Geometry: final body of the model. Coordinates: model frame, mm. A direction names the side the tool comes from. Coordinates: 2 decimals unless noted, no trailing zeros. Order: outer loops, then holes, each group sorted by start corner. A loop starts at its lowest first (then second) coordinate and runs counter-clockwise, first axis right, second up. Notation, with made-up numbers: M 34,-4.75 L 66,-4.75 A20 ccw 66,5.25 Z; hole C 78,-26.5 d2. An arc over 180 degrees is marked long. Use CSV: the item, a comma, the result in double quotes. Start each with the question number.
Q1. Access query for faces 5 (the face through (19.72, 57.1, -140.08)), 6 (the face through (14.58, 202.24, -189)). Directions: +Z, -Z, +X, -X, +Y, -Y. A direction counts if a zero-diameter tool reaches every point of the face in a straight line with its end or side. Return the directions, or none.
Q2. Ray query, probe 1 along X at (y, z) = (4.5, -30); probe 2 along Y at (x, z) = (7.5, -17); probe 3 along Z at (x, y) = (38, 210.5). Return the intervals inside material, ascending.
Q3. First-contact query: P1, Ø7, axis at x = 30, y = 217, coming from the +Z side; P2, Ø10, axis at x = 35.5, y = 45, coming from the -Z side; P3, Ø4, axis at x = 26.5, y = 29.5, coming from the +Z side. Flat tips, straight axial feed; report the tip coordinate or a pass-through.
Q4. Mould query, pull axis Y, two halves, no side actions, for faces 1 (the face through (10.001, 202.684, -184.437)), 2 (the face through (32.027, 7.383, -31.859)), 3 (the face through (23.47, 171.38, -192.04)), 4 (the face through (20, 0, -20)). Classes: +Y half, -Y half, draft (parallel to the pull), parting line (faces both ways), or undercut.
Q5. Section query B-B, the plane y = 187. Output: boundary loops of the cut face in (x, z), and give its area (3 significant figures).
Q6. Section query D-D, the plane y = 39.5. Output: boundary loops of the cut face in (x, z), and give its area (3 significant figures).
Q7. Section query A-A, the plane x = 20. Output: boundary loops of the cut face in (y, z), and give its area (3 significant figures).
Q8. Section query C-C, the plane z = -37. Output: boundary loops of the cut face in (x, y).
from build123d import *

# Parameters (mm, degrees)
BOSS_EXTRUDE2_DEPTH            = 40
M5_CLEARANCE_HOLE2_D           = 5.5
M5_CLEARANCE_HOLE2_CSINK_D     = 5.55
M5_CLEARANCE_HOLE2_CSINK_ANGLE = 90
CUT_EXTRUDE1_REACH             = 303.917
SKETCH10_R                     = 16
SKETCH11_R                     = 18.6
CUT_EXTRUDE2_DEPTH             = 9
FILLET1_START                  = -1
FILLET1_DEPTH                  = 218.778561538
FILLET1_START_2                = -196
FILLET1_2_DEPTH                = 188.2945
M5_CLEARANCE_HOLE3_D           = 5.5
M5_CLEARANCE_HOLE3_CSINK_D     = 5.55
M5_CLEARANCE_HOLE3_CSINK_ANGLE = 90


with BuildPart() as part:
    # Sketch6 → Boss-Extrude2 (new body)
    with BuildSketch(Plane(origin=(0, 0, 0), x_dir=(0, 0, -1), z_dir=(1, 0, 0))):
        with BuildLine():
            Line((0, 0), (40, 0))
            ThreePointArc((40, 0), (149.601551084, 45.398448916), (195, 155))
            Line((195, 155), (195, 227))
            Line((195, 227), (180, 227))
            Line((180, 227), (180, 155))
            ThreePointArc((180, 155), (138.994949366, 56.005050634), (40, 15))
            Line((40, 15), (0, 15))
            Line((0, 15), (0, 0))
        make_face()
    extrude(amount=BOSS_EXTRUDE2_DEPTH)

    # M5 Clearance Hole2 (through all)
    with Locations(Plane(origin=(0, 15, 0), x_dir=(1, 0, 0), z_dir=(0, 1, 0))):
        with Locations((10, 30), (30, 30), (10, 10), (30, 10)):
            CounterSinkHole(M5_CLEARANCE_HOLE2_D / 2, M5_CLEARANCE_HOLE2_CSINK_D / 2, counter_sink_angle=M5_CLEARANCE_HOLE2_CSINK_ANGLE)

    # Sketch10 → Cut-Extrude1 (cut, up to next)
    with BuildSketch(Plane(origin=(0, 0, -195), x_dir=(-1, 0, 0), z_dir=(0, 0, -1)), mode=Mode.PRIVATE) as cut_extrude1_sk1:
        with Locations((-20, 187)):
            Circle(SKETCH10_R)
    cut_extrude1_tool1 = extrude(cut_extrude1_sk1.sketch, amount=-CUT_EXTRUDE1_REACH, mode=Mode.PRIVATE) & part.part
    add(cut_extrude1_tool1.solids().sort_by_distance((20, 187, -195))[0], mode=Mode.SUBTRACT)

    # Sketch11 → Cut-Extrude2 (cut)
    with BuildSketch(Plane(origin=(0, 0, -180), x_dir=(-1, 0, 0), z_dir=(0, 0, -1))):
        with Locations((-20, 187)):
            Circle(SKETCH11_R)
    extrude(amount=CUT_EXTRUDE2_DEPTH, mode=Mode.SUBTRACT)

    # Fillet1: read off the stored shape, not the designer's step
    # Fillet1 outline → Fillet1 (cut)
    with BuildSketch(Plane(origin=(0, 0, 0), x_dir=(1, 0, 0), z_dir=(0, 1, 0)).offset(FILLET1_START)):
        with BuildLine():
            Line((40, 0), (40, 10))
            add(Edge.make_bspline(
                [(40, 10), (40, 0), (30, 0)],
                knots=[0, 0, 0, 1, 1, 1], degree=2, weights=[1, 0.707106781, 1]))
            Line((30, 0), (40, 0))
        make_face()
        with BuildLine():
            Line((0, 0), (10, 0))
            add(Edge.make_bspline(
                [(10, 0), (0, 0), (0, 10)],
                knots=[0, 0, 0, 1, 1, 1], degree=2, weights=[1, 0.707106781, 1]))
            Line((0, 10), (0, 0))
        make_face()
    extrude(amount=FILLET1_DEPTH, mode=Mode.SUBTRACT)

    # Fillet1 2 outline → Fillet1 2 (cut)
    with BuildSketch(Plane.XY.offset(FILLET1_START_2)):
        with BuildLine():
            add(Edge.make_bspline(
                [(10, 227), (0, 227), (0, 217)],
                knots=[0, 0, 0, 1, 1, 1], degree=2, weights=[1, 0.707106781, 1]))
            Line((10, 227), (0, 227))
            Line((0, 227), (0, 217))
        make_face()
        with BuildLine():
            add(Edge.make_bspline(
                [(40, 217), (40, 227), (30, 227)],
                knots=[0, 0, 0, 1, 1, 1], degree=2, weights=[1, 0.707106781, 1]))
            Line((40, 217), (40, 227))
            Line((40, 227), (30, 227))
        make_face()
    extrude(amount=FILLET1_2_DEPTH, mode=Mode.SUBTRACT)

    # M5 Clearance Hole3 (through all)
    with Locations(Plane(origin=(0, 0, -195), x_dir=(-1, 0, 0), z_dir=(0, 0, -1))):
        with Locations((-30, 217), (-10, 217)):
            CounterSinkHole(M5_CLEARANCE_HOLE3_D / 2, M5_CLEARANCE_HOLE3_CSINK_D / 2, counter_sink_angle=M5_CLEARANCE_HOLE3_CSINK_ANGLE)


solid = part.part
Responses:
1,face 5,"+Z, +X, -X, +Y"
1,face 6,"+Z"
2,probe 1,"x = 0 to 7.25, 12.75 to 27.25, 32.75 to 40"
2,probe 2,"y = 0 to 15"
2,probe 3,"z = -195 to -180"
3,P1,"stops at z = -180"
3,P2,"stops at z = -154.02"
3,P3,"stops at z = -97.83"
4,face 1,"undercut"
4,face 2,"draft"
4,face 3,"undercut"
4,face 4,"-Y half"
5,outline,"M 0,-195 L 4,-195 L 4,-189 L 1.4,-189 L 1.4,-180 L 0,-180 Z; M 36,-195 L 40,-195 L 40,-180 L 38.6,-180 L 38.6,-189 L 36,-189 Z"
5,area,"73.2 mm²"
6,outline,"M 0,-143.37 L 40,-143.37 L 40,-119.12 L 0,-119.12 Z"
6,area,"970 mm²"
7,outline,"M 0,-40 A155 ccw 155,-195 L 171,-195 L 171,-189 L 168.4,-189 L 168.4,-180 L 155,-180 A140 cw 15,-40 L 15,0 L 0,0 Z; M 203,-195 L 227,-195 L 227,-180 L 205.6,-180 L 205.6,-189 L 203,-189 Z"
7,area,"4,630 mm²"
8,outline,"M 0,0 L 40,0 L 40,15 L 0,15 Z"
